Source: CAD feature listing. Evaluate the final solid. Frame: model axes, mm. Give positions to 0.01 mm unless a question says otherwise; leave off trailing zeros. Order: outer loops, then holes, each group sorted by start corner. A loop starts at its lowest first (then second) coordinate and runs counter-clockwise, first axis right, second up. Notation, with made-up numbers: M 40,7 L 91,7 A23 cw 91,46 Z; hole C 86,23.5 d5. An arc over 180 degrees is marked long. Answer in a Markdown table with one row per item. Add a question column.
(1) Section query A-A, the plane z = 0. Return loops of the section in (x, y), plus the area to 3 significant figures.
(2) Section query D-D, the plane z = 1.5. Return loops of the section in (x, y), plus the area to 3 significant figures.
(3) Mould query, pull axis Z, two halves, no side actions, for faces 1 (the face through (7.4, -2.15, 0.05)), 2 (the face through (0, -2, 0)), 3 (the face through (0.104, -3.213, 0.714)). Classes: pulls with the +Z half, pulls with the -Z half, needs draft (parallel to the pull), parting line crosses it, or undercut.
(4) Section query B-B, the plane x = -5.5. Return loops of the section in (y, z), plus the area to 3 significant figures.
(5) Pin query (flat end, axial travel): P1, Ø6, axis at x = -5, y = -1, coming from the -Z side; P2, Ø2, axis at y = 7.5, z = 1, coming from the +X side. Return the tip coordinate at first contact, or that it passes through.
(6) Material intervals for line 1 along Y through (x, z) = (1.75, 0); line 2 along X through (y, z) = (11.25, 0.5); line 3 along Y through (x, z) = (-6.5, -1.25), sorted ascending.
(7) Section query C-C, the plane y = 6.75. Return loops of the section in (x, z).
from build123d import *

# Parameters (mm, degrees)
SKETCH_1_R      = 3.291358074
SKETCH_1_R_2    = 2
EXTRUDE_1_DEPTH = 7.4
EXTRUDE_2_DEPTH = 6


with BuildPart() as part:
    # Sketch 1 → Extrude 1 (new, symmetric)
    with BuildSketch(Plane(origin=(0, 0, 0), x_dir=(0, 0, -1), z_dir=(1, 0, 0))):
        Circle(SKETCH_1_R)
        Circle(SKETCH_1_R_2, mode=Mode.SUBTRACT)
    extrude(amount=EXTRUDE_1_DEPTH, both=True)

    # Sketch 1_3 → Extrude 2 (add, symmetric)
    with BuildSketch(Plane(origin=(0, 0, 0), x_dir=(0, 0, -1), z_dir=(1, 0, 0))):
        with BuildLine():
            Line((-3.291358074, 12.376548109), (-3.291358074, 0))
            ThreePointArc((-3.291358074, 0), (0, 3.291358074), (3.291358074, 0))
            Line((3.291358074, 0), (3.291358074, 12.376548109))
            Line((3.291358074, 12.376548109), (-3.291358074, 12.376548109))
        make_face()
    extrude(amount=EXTRUDE_2_DEPTH, both=True)


solid = part.part
Values follow:
| question | item | result |
|---|---|---|
| 1 | outline | M -7.4,-3.29 L 7.4,-3.29 L 7.4,-2 L -7.4,-2 Z; M -7.4,2 L 7.4,2 L 7.4,3.29 L 6,3.29 L 6,12.38 L -6,12.38 L -6,3.29 L -7.4,3.29 Z |
| 1 | area | 147 mm² |
| 2 | outline | M -7.4,-2.93 L 7.4,-2.93 L 7.4,-1.32 L -7.4,-1.32 Z; M -7.4,1.32 L 7.4,1.32 L 7.4,2.93 L 6,2.93 L 6,12.38 L -6,12.38 L -6,2.93 L -7.4,2.93 Z |
| 2 | area | 161 mm² |
| 3 | face 1 | needs draft |
| 3 | face 2 | undercut |
| 3 | face 3 | parting line crosses it |
| 4 | outline | M 0,-3.29 L 12.38,-3.29 L 12.38,3.29 L 0,3.29 A3.29 ccw Z; hole C 0,0 d4 |
| 4 | area | 85.9 mm² |
| 5 | P1 | stops at z = -3.29 |
| 5 | P2 | stops at x = 6 |
| 6 | line 1 | y = -3.29 to -2, 2 to 12.38 |
| 6 | line 2 | x = -6 to 6 |
| 6 | line 3 | y = -3.04 to -1.56, 1.56 to 3.04 |
| 7 | outline | M -6,-3.29 L 6,-3.29 L 6,3.29 L -6,3.29 Z |
